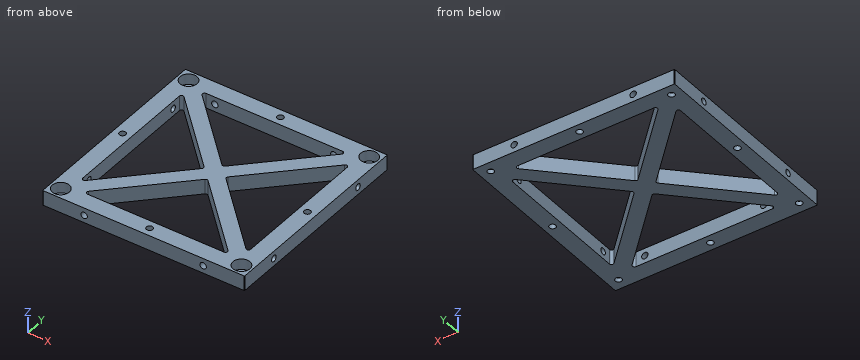
Autodesk Fusion 360 part; units mm, degrees
sketch "Sketch1" plane through (0, 0, 0) normal (0, 0, 1) x (1, 0, 0)
  line L0 (-44.9, 45) -> (49.5, 45)
  line L1 (49.8, 44.7) -> (49.8, -49.7)
  line L2 (49.5, -50) -> (-44.9, -50)
  line L3 (-45.2, -49.7) -> (-45.2, 44.7)
  arc A0 (-44.9, 45) -> (-45.2, 44.7) centre (-44.9, 44.7) ccw
  arc A1 (49.8, 44.7) -> (49.5, 45) centre (49.5, 44.7) ccw
  arc A2 (49.5, -50) -> (49.8, -49.7) centre (49.5, -49.7) ccw
  arc A3 (-45.2, -49.7) -> (-44.9, -50) centre (-44.9, -49.7) ccw
  point P0 (-45.2, 45)
  point P1 (49.8, 45)
  point P2 (-45.2, -50)
  dimension "d1" = 95
  dimension "d2" = 95
  dimension "d3" = 0.3
  dimension "d4" = 0.3
extrude "Extrude1" add sketch "Sketch1" along normal blind 7
sketch "Sketch2" plane through (0, 0, 7) normal (0, 0, 1) x (-1, 0, 0)
  arc A0 (44.9, -45) -> (45.2, -44.7) centre (44.9, -44.7) ccw
  line L0 (45.2, -44.7) -> (45.2, 49.7)
  arc A1 (45.2, 49.7) -> (44.9, 50) centre (44.9, 49.7) ccw
  line L1 (44.9, 50) -> (-49.5, 50)
  arc A2 (-49.5, 50) -> (-49.8, 49.7) centre (-49.5, 49.7) ccw
  line L2 (-49.8, 49.7) -> (-49.8, -44.7)
  arc A3 (-49.8, -44.7) -> (-49.5, -45) centre (-49.5, -44.7) ccw
  line L3 (-49.5, -45) -> (44.9, -45)
  line L4 (-38.8, 42) -> (34.2, 42)
  line L5 (37.2, 39) -> (37.2, -34)
  line L6 (34.2, -37) -> (-38.8, -37)
  line L7 (-41.8, -34) -> (-41.8, 39)
  arc A4 (-41.8, -34) -> (-38.8, -37) centre (-38.8, -34) ccw
  arc A5 (-38.8, 42) -> (-41.8, 39) centre (-38.8, 39) ccw
  arc A6 (37.2, 39) -> (34.2, 42) centre (34.2, 39) ccw
  arc A7 (34.2, -37) -> (37.2, -34) centre (34.2, -34) ccw
  point P0 (-41.8, 42)
  point P1 (37.2, 42)
  point P2 (-41.8, -37)
  dimension "d7" = 79
  dimension "d8" = 79
  dimension "d9" = 8
  dimension "d10" = 8
  dimension "d11" = 3
extrude "Extrude2" cut sketch "Sketch2" against normal blind 10 contours L4 L5 L6 L7 A4 A5 A6 A7
sketch "Sketch3" plane through (0, 0, 7) normal (0, 0, 1) x (-1, 0, 0)
  line L0 (34.2, -37) -> (-38.8, -37)
  arc A0 (-41.8, -34) -> (-38.8, -37) centre (-38.8, -34) ccw
  line L1 (-41.8, -34) -> (-41.8, 39)
  arc A1 (-38.8, 42) -> (-41.8, 39) centre (-38.8, 39) ccw
  line L2 (-38.8, 42) -> (34.2, 42)
  arc A2 (37.2, 39) -> (34.2, 42) centre (34.2, 39) ccw
  line L3 (37.2, 39) -> (37.2, -34)
  arc A3 (34.2, -37) -> (37.2, -34) centre (34.2, -34) ccw
  arc A4 (44.9, -45) -> (45.2, -44.7) centre (44.9, -44.7) ccw
  line L4 (45.2, -44.7) -> (45.2, 49.7)
  arc A5 (45.2, 49.7) -> (44.9, 50) centre (44.9, 49.7) ccw
  line L5 (44.9, 50) -> (-49.5, 50)
  arc A6 (-49.5, 50) -> (-49.8, 49.7) centre (-49.5, 49.7) ccw
  line L6 (-49.8, 49.7) -> (-49.8, -44.7)
  arc A7 (-49.8, -44.7) -> (-49.5, -45) centre (-49.5, -44.7) ccw
  line L7 (-49.5, -45) -> (44.9, -45)
  line L8 (45.2, -45) -> (-49.75, 49.95)
sketch "Sketch4" plane through (0, 0, 7) normal (0, 0, 1) x (-1, 0, 0)
  line L0 (45.2, 50) -> (-49.8, -45)
sketch "Sketch5" plane through (0, 0, 7) normal (0, 0, 1) x (-1, 0, 0)
  line L0 (40.0749, -34.9251) -> (35.1251, -39.8749)
  line L1 (35.1251, -39.8749) -> (-45.1249, 40.3751)
  line L2 (-45.1249, 40.3751) -> (-40.1751, 45.3249)
  line L3 (-40.1751, 45.3249) -> (40.0749, -34.9251)
  line L4 (45.2, -45) -> (-49.75, 49.95)
  dimension "d14" = 3.5
  dimension "d15" = 3.5
extrude "Extrude3" add sketch "Sketch5" against normal blind 7
sketch "Sketch6" plane through (0, 0, 7) normal (0, 0, 1) x (-1, 0, 0)
  line L0 (35.1251, 44.8749) -> (40.0749, 39.9251)
  line L1 (40.0749, 39.9251) -> (-41.1751, -41.3249)
  line L2 (-41.1751, -41.3249) -> (-46.1249, -36.3751)
  line L3 (-46.1249, -36.3751) -> (35.1251, 44.8749)
  line L4 (45.2, 50) -> (-49.8, -45)
  dimension "d18" = 3.5
  dimension "d19" = 3.5
extrude "Extrude4" add sketch "Sketch6" against normal blind 7
sketch "Sketch7" plane through (0, 0, 7) normal (0, 0, 1) x (-1, 0, 0)
  line L0 (37.2, 37.0503) -> (37.2, -32.0503)
  line L1 (37.2, -32.0503) -> (2.6497, 2.5)
  line L2 (2.6497, 2.5) -> (37.2, 37.0503)
  line L3 (-2.3, -2.4497) -> (32.2503, -37)
  line L4 (32.2503, -37) -> (-36.8503, -37)
  line L5 (-36.8503, -37) -> (-2.3, -2.4497)
  line L6 (-7.2497, 2.5) -> (-41.8, -32.0503)
  line L7 (-41.8, -32.0503) -> (-41.8, 37.0503)
  line L8 (-41.8, 37.0503) -> (-7.2497, 2.5)
  line L9 (32.2503, 42) -> (-2.3, 7.4497)
  line L10 (-2.3, 7.4497) -> (-36.8503, 42)
  line L11 (-36.8503, 42) -> (32.2503, 42)
  arc A0 (44.9, -45) -> (45.2, -44.7) centre (44.9, -44.7) ccw
  line L12 (45.2, -44.7) -> (45.2, 49.7)
  arc A1 (45.2, 49.7) -> (44.9, 50) centre (44.9, 49.7) ccw
  line L13 (44.9, 50) -> (-49.5, 50)
  arc A2 (-49.5, 50) -> (-49.8, 49.7) centre (-49.5, 49.7) ccw
  line L14 (-49.8, 49.7) -> (-49.8, -44.7)
  arc A3 (-49.8, -44.7) -> (-49.5, -45) centre (-49.5, -44.7) ccw
  line L15 (-49.5, -45) -> (44.9, -45)
fillet "Fillet1" radius 1 1 edges at (36.8503, -42, 3.5)
fillet "Fillet2" radius 1 1 edges at (41.8, -37.0503, 3.5)
fillet "Fillet3" radius 1 1 edges at (41.8, 32.0503, 3.5)
fillet "Fillet4" radius 1 1 edges at (36.8503, 37, 3.5)
fillet "Fillet5" radius 1 1 edges at (-32.2503, 37, 3.5)
fillet "Fillet6" radius 1 1 edges at (-37.2, 32.0503, 3.5)
fillet "Fillet7" radius 1 1 edges at (-37.2, -37.0503, 3.5)
fillet "Fillet8" radius 1 1 edges at (-32.2503, -42, 3.5)
fillet "Fillet9" radius 1 1 edges at (-2.6497, -2.5, 3.5)
fillet "Fillet10" radius 1 1 edges at (2.3, -7.4497, 3.5)
fillet "Fillet11" radius 1 1 edges at (7.2497, -2.5, 3.5)
fillet "Fillet12" radius 1 1 edges at (2.3, 2.4497, 3.5)
sketch "Sketch8" plane through (0, 0, 7) normal (0, 0, 1) x (-1, 0, 0)
  line L0 (37.2, 34.636) -> (37.2, -29.636)
  arc A0 (35.4929, -30.3431) -> (37.2, -29.636) centre (36.2, -29.636) ccw
  line L1 (35.4929, -30.3431) -> (3.3569, 1.7929)
  arc A1 (3.3569, 3.2071) -> (3.3569, 1.7929) centre (4.064, 2.5) ccw
  line L2 (3.3569, 3.2071) -> (35.4929, 35.3431)
  arc A2 (37.2, 34.636) -> (35.4929, 35.3431) centre (36.2, 34.636) ccw
  arc A3 (29.836, -37) -> (30.5431, -35.2929) centre (29.836, -36) ccw
  line L3 (29.836, -37) -> (-34.436, -37)
  arc A4 (-35.1431, -35.2929) -> (-34.436, -37) centre (-34.436, -36) ccw
  line L4 (-35.1431, -35.2929) -> (-3.0071, -3.1569)
  arc A5 (-1.5929, -3.1569) -> (-3.0071, -3.1569) centre (-2.3, -3.864) ccw
  line L5 (-1.5929, -3.1569) -> (30.5431, -35.2929)
  line L6 (-41.8, -29.636) -> (-41.8, 34.636)
  arc A6 (-40.0929, 35.3431) -> (-41.8, 34.636) centre (-40.8, 34.636) ccw
  line L7 (-40.0929, 35.3431) -> (-7.9569, 3.2071)
  arc A7 (-7.9569, 1.7929) -> (-7.9569, 3.2071) centre (-8.664, 2.5) ccw
  line L8 (-7.9569, 1.7929) -> (-40.0929, -30.3431)
  arc A8 (-41.8, -29.636) -> (-40.0929, -30.3431) centre (-40.8, -29.636) ccw
  line L9 (-3.0071, 8.1569) -> (-35.1431, 40.2929)
  arc A9 (-34.436, 42) -> (-35.1431, 40.2929) centre (-34.436, 41) ccw
  line L10 (-34.436, 42) -> (29.836, 42)
  arc A10 (30.5431, 40.2929) -> (29.836, 42) centre (29.836, 41) ccw
  line L11 (30.5431, 40.2929) -> (-1.5929, 8.1569)
  arc A11 (-3.0071, 8.1569) -> (-1.5929, 8.1569) centre (-2.3, 8.864) ccw
  arc A12 (44.9, -45) -> (45.2, -44.7) centre (44.9, -44.7) ccw
  line L12 (45.2, -44.7) -> (45.2, 49.7)
  arc A13 (45.2, 49.7) -> (44.9, 50) centre (44.9, 49.7) ccw
  line L13 (44.9, 50) -> (-49.5, 50)
  arc A14 (-49.5, 50) -> (-49.8, 49.7) centre (-49.5, 49.7) ccw
  line L14 (-49.8, 49.7) -> (-49.8, -44.7)
  arc A15 (-49.8, -44.7) -> (-49.5, -45) centre (-49.5, -44.7) ccw
  line L15 (-49.5, -45) -> (44.9, -45)
  line L16 (44.9, 50) -> (-49.5, 50)
  line L17 (-49.5, -45) -> (44.9, -45)
  point P0 (40.2, 45)
  point P1 (-44.8, 45)
  point P2 (40.2, -40)
  point P3 (-44.8, -40)
  dimension "d46" = 5
  dimension "d47" = 5
  dimension "d48" = 5
  dimension "d49" = 5
  dimension "d50" = 5
  dimension "d51" = 5
  dimension "d52" = 5
  dimension "d53" = 5
hole "Hole1" at (44.8, 40, 7) at (-40.2, 40, 7) at (-40.2, -45, 7) at (44.8, -45, 7) direction (0, 0, -1) diameter 3 depth 15 tip angle 118
sketch "Sketch9" plane through (0, 0, 7) normal (0, 0, 1) x (-1, 0, 0)
  circle A0 centre (40.2, -40) radius 4
  line L0 (45.2, -44.7) -> (45.2, 49.7)
  line L1 (-49.5, -45) -> (44.9, -45)
  circle A1 centre (-44.8, -40) radius 4
  line L2 (-49.8, 49.7) -> (-49.8, -44.7)
  circle A2 centre (-44.8, 45) radius 4
  line L3 (44.9, 50) -> (-49.5, 50)
  circle A3 centre (40.2, 45) radius 4
  dimension "d57" = 8
  dimension "d58" = 5
  dimension "d59" = 5
  dimension "d60" = 8
  dimension "d61" = 5
  dimension "d62" = 5
  dimension "d63" = 8
  dimension "d64" = 5
  dimension "d65" = 5
  dimension "d66" = 8
  dimension "d67" = 5
  dimension "d68" = 5
extrude "Extrude5" cut sketch "Sketch9" against normal blind 5
sketch "Sketch10" plane through (0, 0, 7) normal (0, 0, 1) x (-1, 0, 0)
  line L0 (45.2, -44.7) -> (45.2, 49.7)
  line L1 (-49.5, -45) -> (44.9, -45)
  line L2 (-49.8, 49.7) -> (-49.8, -44.7)
  line L3 (44.9, 50) -> (-49.5, 50)
  point P0 (-2.3, -41)
  point P1 (41.2, 2.5)
  point P2 (-2.3, 46)
  point P3 (-45.8, 2.5)
  dimension "d71" = 4
  dimension "d72" = 47.5
  dimension "d73" = 4
  dimension "d74" = 47.5
  dimension "d75" = 4
  dimension "d76" = 47.5
  dimension "d77" = 4
  dimension "d78" = 47.5
hole "Hole2" at (2.3, -46, 7) at (-41.2, -2.5, 7) at (45.8, -2.5, 7) at (2.3, 41, 7) direction (0, 0, -1) diameter 3 depth 15 tip angle 118
sketch "Sketch11" plane through (0, -50, 0) normal (0, -1, 0) x (1, 0, 0)
  line L0 (-44.9, 0) -> (49.5, 0)
  line L1 (49.5, 0) -> (49.5, 7)
  line L2 (49.5, 7) -> (-44.9, 7)
  line L3 (-44.9, 7) -> (-44.9, 0)
  line L4 (49.8, 0) -> (49.8, 7)
  point P0 (-25.7, 3.5)
  point P1 (2.3, 3.5)
  point P2 (30.3, 3.5)
  dimension "d82" = 3.5
  dimension "d83" = 28
  dimension "d84" = 28
  dimension "d85" = 47.5
  dimension "d86" = 3.5
  dimension "d87" = 3.5
hole "Hole3" at (-25.7, -50, 3.5) at (30.3, -50, 3.5) direction (0, 1, 0) diameter 3 depth 11 tip angle 118
sketch "Sketch12" plane through (49.8, 0, 0) normal (1, 0, 0) x (0, 1, 0)
  line L0 (-49.7, 0) -> (44.7, 0)
  line L1 (44.7, 0) -> (44.7, 7)
  line L2 (44.7, 7) -> (-49.7, 7)
  line L3 (-49.7, 7) -> (-49.7, 0)
  line L4 (-50, 0) -> (-50, 7)
  point P0 (-30.5, 3.5)
  point P1 (-2.5, 3.5)
  point P2 (25.5, 3.5)
  dimension "d91" = 47.5
  dimension "d92" = 28
  dimension "d93" = 28
  dimension "d94" = 3.5
  dimension "d95" = 3.5
  dimension "d96" = 3.5
hole "Hole4" at (49.8, -30.5, 3.5) at (49.8, 25.5, 3.5) direction (-1, 0, 0) diameter 3 depth 11 tip angle 118
sketch "Sketch13" plane through (0, 0, 7) normal (0, 0, 1) x (1, 0, 0)
sketch "Sketch14" plane through (0, 45, 0) normal (0, 1, 0) x (-1, 0, 0)
  line L0 (-49.5, 0) -> (44.9, 0)
  line L1 (44.9, 0) -> (44.9, 7)
  line L2 (44.9, 7) -> (-49.5, 7)
  line L3 (-49.5, 7) -> (-49.5, 0)
  line L4 (-49.8, 0) -> (-49.8, 7)
  point P0 (-30.3, 3.5)
  point P1 (-2.3, 3.5)
  point P2 (25.7, 3.5)
  dimension "d100" = 47.5
  dimension "d101" = 28
  dimension "d102" = 28
  dimension "d103" = 3.5
  dimension "d104" = 3.5
  dimension "d105" = 3.5
hole "Hole5" at (30.3, 45, 3.5) at (-25.7, 45, 3.5) direction (0, -1, 0) diameter 3 depth 11 tip angle 118
sketch "Sketch15" plane through (-45.2, 0, 0) normal (-1, 0, 0) x (0, -1, 0)
  line L0 (-44.7, 0) -> (49.7, 0)
  line L1 (49.7, 0) -> (49.7, 7)
  line L2 (49.7, 7) -> (-44.7, 7)
  line L3 (-44.7, 7) -> (-44.7, 0)
  line L4 (-45, 0) -> (-45, 7)
  point P0 (-25.5, 3.5)
  point P1 (2.5, 3.5)
  point P2 (30.5, 3.5)
  dimension "d109" = 47.5
  dimension "d110" = 28
  dimension "d111" = 28
  dimension "d112" = 3.5
  dimension "d113" = 3.5
  dimension "d114" = 3.5
hole "Hole6" at (-45.2, 25.5, 3.5) at (-45.2, -30.5, 3.5) direction (1, 0, 0) diameter 3 depth 11 tip angle 118
Design review of the part built by this model. Coordinates are the model's own, in mm. Round coordinates to 2 decimals unless told otherwise and drop trailing zeros. Order: outer loops, then holes, each group sorted by start corner. A loop starts at its lowest first (then second) coordinate and runs counter-clockwise, first axis right, second up. Notation, with made-up numbers: M 71,-34 L 129,-34 A30 ccw 129,3 Z; hole C -19.5,59.25 d7. An arc over 180 degrees is marked long. Answer as CSV lines item,"result". Start each with the question number.
1) Add section C-C (x = -13). Give the boundary of the cut face in (y, z).
2) Add section A-A (x = -25.7). Give the boundary of the cut face in (y, z).
3) For pin 1 Ø5 at (x, y) = (44.8, 40) entering from +Z; pin 2 Ø2.5 at (y, z) = (-30.5, 3.5) entering from -X, all flat-tipped, find the tip position at first contact; note any pin that passes through.
4) Wall thickness on line 1 along Y through (x, z) = (2.3, 2); line 2 along Y through (x, z) = (45.5, 2.75); line 3 along Y through (x, z) = (12, 2.25): over which ranges is each line inside the solid? List them lowest first. Write a range as [from, to].
5) Add section D-D (y = -11). Give the boundary of the cut face in (x, z), then the cut area to 3 significant figures.
6) Add section B-B (y = -30.5). Give the boundary of the cut face in (x, z).
Resolved:
1,outline,"M -50,0 L -42,0 L -42,7 L -50,7 Z; M -22.75,0 L -12.85,0 L -12.85,7 L -22.75,7 Z; M 7.85,0 L 17.75,0 L 17.75,7 L 7.85,7 Z; M 37,0 L 45,0 L 45,7 L 37,7 Z"
2,outline,"M -50,0 L -42,0 L -42,2 L -50,2 Z; M -50,5 L -42,5 L -42,7 L -50,7 Z; M -35.45,0 L -25.55,0 L -25.55,7 L -35.45,7 Z; M 20.55,0 L 30.45,0 L 30.45,7 L 20.55,7 Z; M 37,0 L 45,0 L 45,2 L 37,2 Z; M 37,5 L 45,5 L 45,7 L 37,7 Z"
3,pin 1,"z = 2"
3,pin 2,"x = -31.9"
4,line 1,"[-50, -47.5], [-44.5, -42], [-7.86, 2.86], [37, 39.5], [42.5, 45]"
4,line 2,"[-50, -48.94], [-41.06, -31.8], [-29.2, -3.97], [-1.03, 24.2], [26.8, 36.06], [43.94, 45]"
4,line 3,"[-50, -42], [-17.15, -7.25], [2.25, 12.15], [37, 45]"
5,outline,"M -45.2,0 L -37.2,0 L -37.2,7 L -45.2,7 Z; M -11.15,0 L -1.25,0 L -1.25,7 L -11.15,7 Z; M 5.85,0 L 15.75,0 L 15.75,7 L 5.85,7 Z; M 41.8,0 L 49.8,0 L 49.8,7 L 41.8,7 Z"
5,area,"251 mm^2"
6,outline,"M -45.2,0 L -37.2,0 L -37.2,2 L -45.2,2 Z; M -45.2,5 L -37.2,5 L -37.2,7 L -45.2,7 Z; M -30.65,0 L -20.75,0 L -20.75,7 L -30.65,7 Z; M 25.35,0 L 35.25,0 L 35.25,7 L 25.35,7 Z; M 41.8,0 L 49.8,0 L 49.8,2 L 41.8,2 Z; M 41.8,5 L 49.8,5 L 49.8,7 L 41.8,7 Z"
